The model under review builds one solid part; all positions refer to its coordinate system, in mm. Face numbers are marked on the shaded views. A direction names the side the tool comes from. Round coordinates to 2 decimals unless told otherwise and drop trailing zeros. Loops run counter-clockwise (first coordinate to the right, second up) from the corner with the lowest first, then second, coordinate; pieces in that order, holes last. Notation, with made-up numbers: (-17, 70.25) -> (36, 70.25) arc R17 ccw to (36, 101.25) -> close; hole circle Ø2 at (59, 1.5). An arc over 180 degrees is marked (long way). Use a Markdown table: item, result. Add a question column.
1) Consider section A-A on x = 0. Give the boundary of the cut face in (y, z), plus the area to 3 significant figures.
2) Consider section C-C on y = 779.5. Give the boundary of the cut face in (x, z), plus the area to 3 significant figures.
3) Consider section D-D on y = 271. Give the boundary of the cut face in (x, z).
4) Consider section B-B on z = 0. Give the boundary of the cut face in (x, y).
5) Insertion check: pin 1 (2 mm diameter, centred on x = 13.5, y = 254.5, fed in from +Z); pin 2 (2 mm diameter, centred on x = -10.5, y = 639, fed in from +Z); pin 3 (1.5 mm diameter, centred on x = 2, y = 264, fed in from -Z). Each pin has a flat end and moves straight along its axis. Give the tip position at first contact, or say it passes through.
6) Wall thickness on probe 1 along Z at (x, y) = (2.5, 106); probe 2 along Y at (x, z) = (-12, -15); probe 3 along Z at (x, y) = (0.5, 180): over which ranges is each line inside the solid? List them lowest first.
7) For the marked faces 1, 2 and 3, list the 3-axis set-ups (+Z, -Z, +X, -X, +Y, -Y) from which the entire face can be reached by the end or side of a thin tool; tool diameter is ignored.
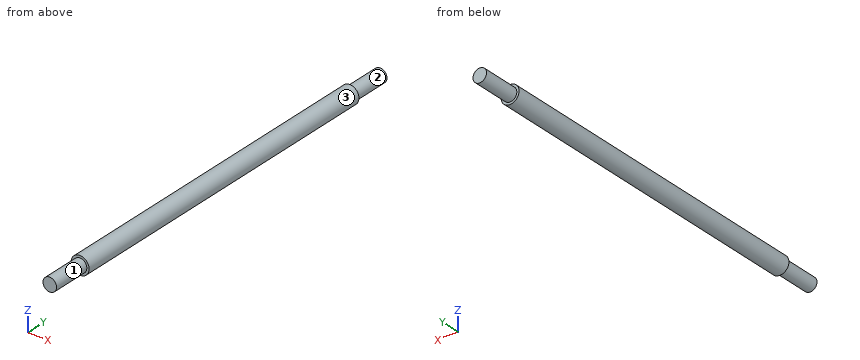
from build123d import *

# Parameters (mm, degrees)
F0_R     = 20
F1_DEPTH = 757
F2_R     = 15
F4_DEPTH = 85
F3_R     = 15
F5_DEPTH = 85


with BuildPart() as f1:
    # F0 (on Front) → F1 (new body)
    with BuildSketch(Plane.XZ):
        Circle(F0_R)
    extrude(amount=-F1_DEPTH)

    # F2 (on face) → F4 (join)
    with BuildSketch(Plane.XZ):
        Circle(F2_R)
    extrude(amount=F4_DEPTH)

    # F3 (on face) → F5 (join)
    with BuildSketch(Plane(origin=(0, 757, 0), x_dir=(-1, 0, 0), z_dir=(0, 1, 0))):
        Circle(F3_R)
    extrude(amount=F5_DEPTH)


solid = f1.part
Result set:
| question | item | result |
|---|---|---|
| 1 | outline | (-85, -15) -> (0, -15) -> (0, -20) -> (757, -20) -> (757, -15) -> (842, -15) -> (842, 15) -> (757, 15) -> (757, 20) -> (0, 20) -> (0, 15) -> (-85, 15) -> close |
| 1 | area | 35,400 mm2 |
| 2 | outline | circle Ø30 at (0, 0) |
| 2 | area | 707 mm2 |
| 3 | outline | circle Ø40 at (0, 0) |
| 4 | outline | (-20, 0) -> (-15, 0) -> (-15, -85) -> (15, -85) -> (15, 0) -> (20, 0) -> (20, 757) -> (15, 757) -> (15, 842) -> (-15, 842) -> (-15, 757) -> (-20, 757) -> close |
| 5 | pin 1 | z = 15.61 |
| 5 | pin 2 | z = 17.6 |
| 5 | pin 3 | z = -19.96 |
| 6 | probe 1 | -19.84 to 19.84 |
| 6 | probe 2 | 0 to 757 |
| 6 | probe 3 | -19.99 to 19.99 |
| 7 | face 1 | -Y |
| 7 | face 2 | +Y |
| 7 | face 3 | +Y, -Y |
